```python
from build123d import *

# Parameters (mm, degrees)
SCHIZZO13_R                  = 1.5
SCHIZZO13_R_2                = 2.75
ESTRUSIONE_ESTRUSIONE2_DEPTH = 6


with BuildPart() as part:
    # Schizzo13 → Estrusione-Estrusione2 (new body)
    with BuildSketch(Plane.XY):
        with BuildLine():
            Line((10, 0), (24.28195797, 0))
            Line((24.28195797, 0), (34.28195797, 10))
            Line((34.28195797, 10), (34.28195797, 30))
            Line((34.28195797, 30), (57.017366293, 53.192694567))
            Line((57.017366293, 53.192694567), (83.745372993, 53.192694567))
            Line((83.745372993, 53.192694567), (107.404551383, 30))
            Line((107.404551383, 30), (107.404551383, 10))
            Line((107.404551383, 10), (117.404551383, 0))
            Line((117.404551383, 0), (232.595448617, 0))
            Line((232.595448617, 0), (242.595448617, 10))
            Line((242.595448617, 10), (242.595448617, 30))
            Line((242.595448617, 30), (266.254627007, 53.192694567))
            Line((266.254627007, 53.192694567), (292.982633707, 53.192694567))
            Line((292.982633707, 53.192694567), (315.71804203, 30))
            Line((315.71804203, 30), (315.71804203, 10))
            Line((315.71804203, 10), (325.71804203, 0))
            Line((325.71804203, 0), (340, 0))
            Line((340, 0), (350, 10))
            Line((350, 10), (350, 70.5))
            Line((350, 70.5), (292.919241786, 124.388863529))
            Line((292.919241786, 124.388863529), (292.919241786, 225.611136471))
            Line((292.919241786, 225.611136471), (350, 279.5))
            Line((350, 279.5), (350, 340))
            Line((350, 340), (340, 350))
            Line((340, 350), (302.982633707, 350))
            Line((302.982633707, 350), (292.982633707, 340))
            Line((292.982633707, 340), (292.982633707, 299.807305433))
            ThreePointArc((292.982633707, 299.807305433), (292.103954051, 297.685985089), (289.982633707, 296.807305433))
            Line((289.982633707, 296.807305433), (266.254627007, 296.807305433))
            Line((266.254627007, 296.807305433), (242.595448617, 320))
            Line((242.595448617, 320), (242.595448617, 340))
            Line((242.595448617, 340), (232.595448617, 350))
            Line((232.595448617, 350), (117.404551383, 350))
            Line((117.404551383, 350), (107.404551383, 340))
            Line((107.404551383, 340), (107.404551383, 320))
            Line((107.404551383, 320), (83.745372993, 296.807305433))
            Line((83.745372993, 296.807305433), (57.017366293, 296.807305433))
            Line((57.017366293, 296.807305433), (34.28195797, 320))
            Line((34.28195797, 320), (34.28195797, 340))
            Line((34.28195797, 340), (24.28195797, 350))
            Line((24.28195797, 350), (10, 350))
            Line((10, 350), (0, 340))
            Line((0, 340), (0, 279.5))
            Line((0, 279.5), (57.080758214, 225.611136471))
            Line((57.080758214, 225.611136471), (57.080758214, 175))
            Line((57.080758214, 175), (57.080758214, 124.388863529))
            Line((57.080758214, 124.388863529), (0, 70.5))
            Line((0, 70.5), (0, 10))
            Line((0, 10), (10, 0))
        make_face()
        with Locations((15, 320)):
            Circle(SCHIZZO13_R, mode=Mode.SUBTRACT)
        with Locations((20.5, 279.5)):
            Circle(SCHIZZO13_R, mode=Mode.SUBTRACT)
        with Locations((57.080758214, 279.5)):
            Circle(SCHIZZO13_R, mode=Mode.SUBTRACT)
        with Locations((175, 175)):
            Circle(SCHIZZO13_R, mode=Mode.SUBTRACT)
        with Locations((20.5, 70.5)):
            Circle(SCHIZZO13_R, mode=Mode.SUBTRACT)
        with Locations((200, 344)):
            Circle(SCHIZZO13_R_2, mode=Mode.SUBTRACT)
        with Locations(Location((150, 344, 0), (0, 0, 180))):
            Circle(SCHIZZO13_R_2, mode=Mode.SUBTRACT)
        with Locations((175, 329)):
            Circle(SCHIZZO13_R_2, mode=Mode.SUBTRACT)
        with Locations((217, 329)):
            Circle(SCHIZZO13_R_2, mode=Mode.SUBTRACT)
        with Locations(Location((133, 329, 0), (0, 0, 180))):
            Circle(SCHIZZO13_R_2, mode=Mode.SUBTRACT)
        with Locations((70.5, 70.5)):
            Circle(SCHIZZO13_R, mode=Mode.SUBTRACT)
        with Locations((279.5, 70.5)):
            Circle(SCHIZZO13_R, mode=Mode.SUBTRACT)
        with Locations((329.5, 70.5)):
            Circle(SCHIZZO13_R, mode=Mode.SUBTRACT)
        with Locations((335, 10)):
            Circle(SCHIZZO13_R, mode=Mode.SUBTRACT)
        with Locations((15, 10)):
            Circle(SCHIZZO13_R, mode=Mode.SUBTRACT)
        with Locations((279.5, 279.5)):
            Circle(SCHIZZO13_R, mode=Mode.SUBTRACT)
        with Locations((329.5, 279.5)):
            Circle(SCHIZZO13_R, mode=Mode.SUBTRACT)
        with Locations((335, 320)):
            Circle(SCHIZZO13_R, mode=Mode.SUBTRACT)
        with Locations((310, 344)):
            Circle(SCHIZZO13_R, mode=Mode.SUBTRACT)
        with Locations((330, 344)):
            Circle(SCHIZZO13_R, mode=Mode.SUBTRACT)
        Polygon((217, 193.286910978), (227.343033378, 225.611136471), (185.750894453, 266.383210572), (164.249105547, 266.383210572), (122.656966622, 225.611136471), (133, 193.286910978), align=None, mode=Mode.SUBTRACT)
        Polygon((133, 156.713089022), (101.348199345, 83.616789428), (155.254193112, 30), (194.745806888, 30), (248.651800655, 83.616789428), (217, 156.713089022), align=None, mode=Mode.SUBTRACT)
    extrude(amount=-ESTRUSIONE_ESTRUSIONE2_DEPTH)


solid = part.part
```
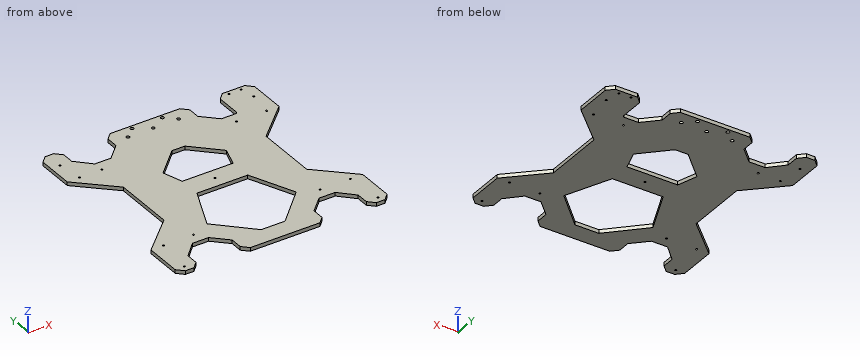
Verification items for the finished model (mm, model axes). Round coordinates to 2 decimals unless told otherwise and drop trailing zeros. Order: outer loops, then holes, each group sorted by start corner. A loop starts at its lowest first (then second) coordinate and runs counter-clockwise, first axis right, second up. Notation, with made-up numbers: (-16.75, -31.5) -> (5.25, -31.5) arc R19 cw to (5.25, -9.5) -> close; hole circle Ø11 at (53, 42.25). An arc over 180 degrees is marked (long way). Put each result on its own line as item: value. Start each with the question number.
(1) Section check D-D (x = 255.5). Enter the section's corners in (y, z).
(2) Section check C-C (y = 166.5). Enter the section's corners in (x, z).
(3) Section check A-A (y = 250). Enter the section's corners in (x, z).
(4) Depth check by flat-ended pin: pin 1 Ø3.5 at (x, y) = (217, 329) entering from +Z; pin 2 Ø1.8 at (x, z) = (74.5, -2.5) entering from -Y. Enter the tip coordinate at first touch or a pass-through.
(5) Material ranges on line 1 along Y through (x, z) = (164.5, -2.35); line 2 along X through (y, z) = (333.5, -1.9); line 3 along Y through (x, z) = (177, -1.05), recorded low to high.
(6) Section check B-B (z = -3.9). State how many separate pieces and enclosed holes the cut face has, then the cut area to 3 significant figures.
Completed:
1. outline: (42.65, -6) -> (307.35, -6) -> (307.35, 0) -> (42.65, 0) -> close
2. outline: (57.08, -6) -> (292.92, -6) -> (292.92, 0) -> (57.08, 0) -> close
3. outline: (31.25, -6) -> (147.54, -6) -> (147.54, 0) -> (31.25, 0) -> close; (202.46, -6) -> (318.75, -6) -> (318.75, 0) -> (202.46, 0) -> close
4. pin 1: passes through
4. pin 2: stops at y = 53.19
5. line 1: y = 0 to 30, 156.71 to 193.29, 266.38 to 350
5. line 2: x = 0 to 34.28, 107.4 to 242.6, 292.98 to 350
5. line 3: y = 0 to 30, 156.71 to 193.29, 266.38 to 327.11, 330.89 to 350
6. separate pieces: 1
6. enclosed holes: 22
6. area: 72,400 mm2
